Answer from the drawing. Dimensions are ordinates in mm from the lowest x, y and z of the part. A direction names the side the tool comes from. Give positions to 0.01 mm unless a question says otherwise; leave off trailing zeros. Write each loop counter-clockwise with the first axis right and the second up, starting at its lowest first coordinate (ties: lowest second). Pieces come first, ordered by that corner, then holes.
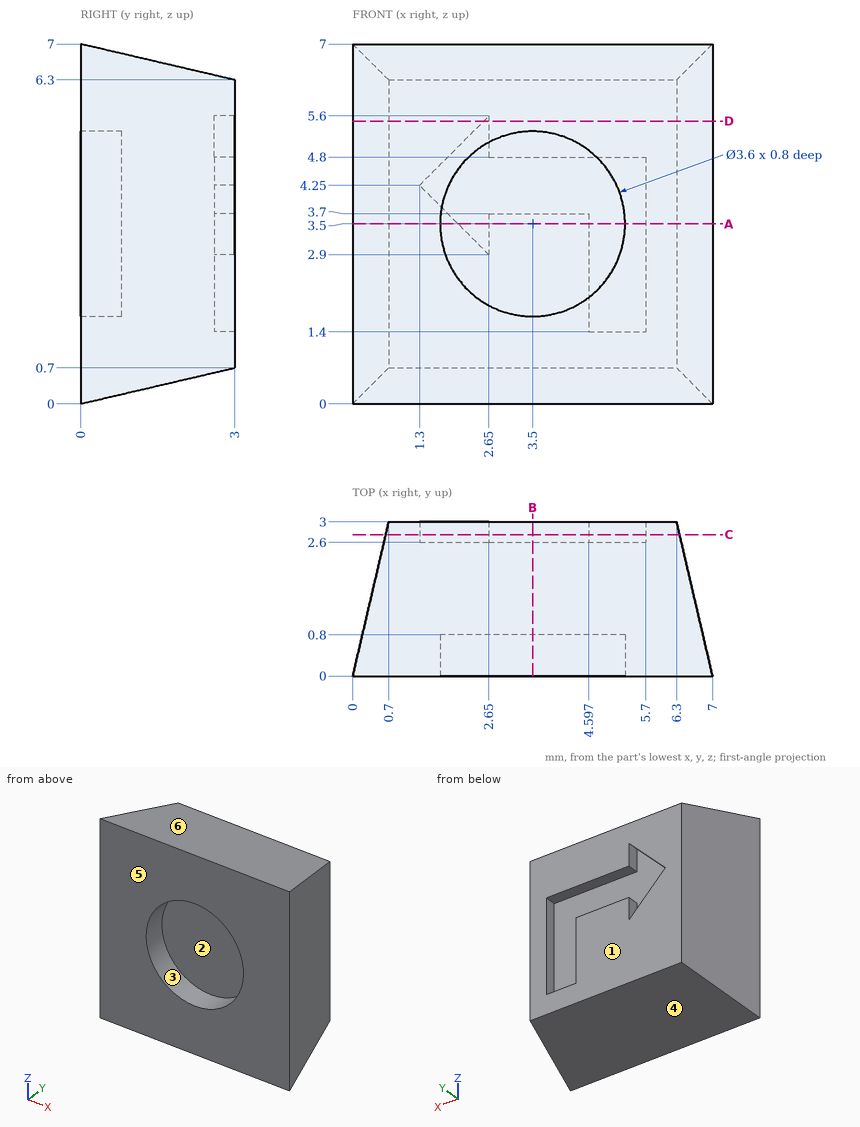
Item 1: Section C-C (y = 2.75) is taken. Write down the section's boundary in (x, z).
Result set:
outline: (0.64, 0.64) - (6.36, 0.64) - (6.36, 6.36) - (0.64, 6.36) - close; hole (1.3, 4.25) - (2.65, 2.9) - (2.65, 3.7) - (4.6, 3.7) - (4.6, 1.4) - (5.7, 1.4) - (5.7, 4.8) - (2.65, 4.8) - (2.65, 5.6) - close
Item 2: Find the intervals of material crossed by line 1 along X through (y, z) = (0.6, 3.5); line 2 along X through (y, z) = (2.7, 2.25); line 3 along Y through (x, z) = (3, 4.75), in increasing order.
Result set:
line 1: x = 0.14 to 1.7, 5.3 to 6.86
line 2: x = 0.63 to 4.6, 5.7 to 6.37
line 3: y = 0.8 to 2.6
Item 3: Determine the mould class of the marked faces 3, 4, 5 and 6 for opening direction Z: pulls with the +Z half, pulls with the -Z half, needs draft (parallel to the pull), parting line crosses it, or undercut.
Result set:
face 3: undercut
face 4: pulls with the -Z half
face 5: needs draft
face 6: pulls with the +Z half
Item 4: Which of the six approach directions +Z, -Z, +X, -X, +Y, -Y give full straight-line access (tool end or side, diameter ignored) to the marked faces 1 and 2?
Result set:
face 1: +Z, -Z, +X, -X, +Y
face 2: -Y
Item 5: Section B-B (x = 3.5) is taken. Write down the section's boundary in (y, z), and give its area (3 significant figures).
Result set:
outline: (0, 0) - (3, 0.7) - (3, 3.7) - (2.6, 3.7) - (2.6, 4.8) - (3, 4.8) - (3, 6.3) - (0, 7) - (0, 5.3) - (0.8, 5.3) - (0.8, 1.7) - (0, 1.7) - close
area: 15.6 mm2
Item 6: Each of these flat-tipped pins is pushed along its axis until it touches: pin 1 Ø3 at (x, z) = (3.5, 3.5) entering from -Y; pin 2 Ø1.5 at (y, z) = (1, 4) entering from -X. Where does it stop, or does it pass through?
Result set:
pin 1: stops at y = 0.8
pin 2: stops at x = 0.06
Item 7: Section A-A (z = 3.5) is taken. Write down the section's boundary in (x, y).
Result set:
outline: (0, 0) - (1.7, 0) - (1.7, 0.8) - (5.3, 0.8) - (5.3, 0) - (7, 0) - (6.3, 3) - (5.7, 3) - (5.7, 2.6) - (4.6, 2.6) - (4.6, 3) - (2.65, 3) - (2.65, 2.6) - (2.05, 2.6) - (2.05, 3) - (0.7, 3) - close
Item 8: Section D-D (z = 5.5) is taken. Write down the section's boundary in (x, y).
Result set:
outline: (0, 0) - (7, 0) - (6.3, 3) - (2.65, 3) - (2.65, 2.6) - (2.55, 2.6) - (2.55, 3) - (0.7, 3) - close
